Read the model definition and answer for the solid it produces. Units are mm, in the model's axes. A direction names the side the tool comes from. Round coordinates to 2 decimals unless told otherwise and drop trailing zeros. Loops run counter-clockwise (first coordinate to the right, second up) from the corner with the lowest first, then second, coordinate; pieces in that order, holes last. Notation, with made-up numbers: M -0.5,29 L 22.5,29 A26 cw 22.5,62 Z; hole C 23,1 d5. An arc over 180 degrees is marked long. Write each question's results on one line, items separated by ' | '.
Autodesk Inventor part; units mm, degrees
ref_plane "YZ Plane" through (0, 0, 0) normal (1, 0, 0) x (0, 1, 0)
ref_plane "XZ Plane" through (0, 0, 0) normal (0, 1, 0) x (-1, 0, 0)
ref_plane "XY Plane" through (0, 0, 0) normal (0, 0, 1) x (1, 0, 0)
sketch "Sketch1" plane through (0, 0, 0) normal (0, 0, 1) x (1, 0, 0)
  circle A0 centre (0, 0) radius 14
  circle A1 centre (0, 0) radius 20
  circle A2 centre (0, 0) radius 26
  circle A3 centre (0, 0) radius 31
  circle A4 centre (0, 0) radius 49
  circle A5 centre (0, 38.5) radius 7
  circle A6 centre (0, 38.5) radius 4
  dimension "d0" = 28
  dimension "d1" = 40
  dimension "d2" = 52
  dimension "d3" = 62
  dimension "d4" = 98
  dimension "d5" = 14
  dimension "d6" = 8
  dimension "d7" = 38.5
extrude "Extrusion1" add sketch "Sketch1" along normal blind 27.25 contours A0 | A1 | A2 | A3 | A4 | A5 | A6
extrude "Extrusion2" cut sketch "Sketch1" along normal through all contours A0
extrude "Extrusion3" cut sketch "Sketch1" along normal blind 7.25 contours A4 | A5 | A6
extrude "Extrusion4" cut sketch "Sketch1" along normal through all contours A6
extrude "Extrusion5" cut sketch "Sketch1" against normal blind 8 from surface at 27.25 contours A5
pattern_circular "Circular Pattern1" count 6 over 360 about axis through (0, 0, -10) along (0, 0, 1) of "Extrusion5", "Extrusion4"
extrude "Extrusion6" cut sketch "Sketch1" along normal blind 10 contours A0 | A1 | A2
extrude "Extrusion7" cut sketch "Sketch1" along normal blind 10 from surface at 10 contours A1
properties part number "B2"
Item 1: Straight lines are drawn through the part: line 1 (Y direction, x = 0, z = 23); line 2 (Y direction, x = 0, z = 13.5); line 3 (Y direction, x = -27.5, z = 21.25). For each, find the intervals that lie inside material, in ascending order.
Outcome:
line 1: y = -49 to -45.5, -31.5 to -14, 14 to 31.5, 45.5 to 49 | line 2: y = -49 to -42.5, -34.5 to -20, 20 to 34.5, 42.5 to 49 | line 3: y = -40.56 to -23.11, -15.39 to 15.39, 23.11 to 40.56
Item 2: The mould has two halves that part along Y. Classify faces 4 (the face through (-32, -15, 19.25)), 5 (the face through (26.34, -41.32, 17.11)), 6 (the face through (3, 35, 19.25)), 7 (the face through (10.2, -10.2, 27.25)): pulls with the +Y half, pulls with the -Y half, needs draft (parallel to the pull), parting line crosses it, or undercut.
Outcome:
face 4: undercut | face 5: parting line crosses it | face 6: undercut | face 7: needs draft
Item 3: The part is cut by section C-C (x = -9.5). Determine the outline of the cut face in (y, z), plus the area to 3 significant figures.
Outcome:
outline: M -48.07,7.25 L -29.51,7.25 L -29.51,0 L -24.2,0 L -24.2,10 L -17.6,10 L -17.6,20 L -10.28,20 L -10.28,27.25 L -48.07,27.25 Z; M 10.28,20 L 17.6,20 L 17.6,10 L 24.2,10 L 24.2,0 L 29.51,0 L 29.51,7.25 L 48.07,7.25 L 48.07,27.25 L 10.28,27.25 Z | area: 1,370 mm2
Item 4: Flat-ended cylindrical pins translate along their axes: pin 1 (6.5 mm diameter, centred on x = 33.34, y = 19.25, fed in from -Z); pin 2 (10 mm diameter, centred on x = 28, z = 4, fed in from -Y); pin 3 (9 mm diameter, centred on x = 33.34, y = -19.25, fed in from +Z); pin 4 (9 mm diameter, centred on x = -33.34, y = -19.25, fed in from -Z). Find the tip coordinate at first contact, or state that the pin passes through.
Outcome:
pin 1: passes through | pin 2: stops at y = -42.61 | pin 3: stops at z = 19.25 | pin 4: stops at z = 7.25
Item 5: For faces 1 (the face through (13.4, -15.3, 10)), 2 (the face through (-0.521, 34.534, 13.166)), 3 (the face through (-3, -35, 19.25)), determine the directions among +Z, -Z, +X, -X, +Y, -Y from which every point of the face is accessible in a straight line to the end or side of a thin tool.
Outcome:
face 1: -Z | face 2: +Z, -Z | face 3: +Z
Item 6: The part is cut by section A-A (y = 0). Determine the outline of the cut face in (x, z), plus the area to 3 significant figures.
Outcome:
outline: M -49,7.25 L -31,7.25 L -31,0 L -26,0 L -26,10 L -20,10 L -20,20 L -14,20 L -14,27.25 L -49,27.25 Z; M 14,20 L 20,20 L 20,10 L 26,10 L 26,0 L 31,0 L 31,7.25 L 49,7.25 L 49,27.25 L 14,27.25 Z | area: 1,290 mm2
Item 7: The part is cut by section D-D (z = 24.5). Determine the outline of the cut face in (x, y).
Outcome:
outline: C 0,0 d98; hole C -33.34,-19.25 d14; hole C -33.34,19.25 d14; hole C 0,0 d28; hole C 0,-38.5 d14; hole C 0,38.5 d14; hole C 33.34,-19.25 d14; hole C 33.34,19.25 d14
Item 8: The part is cut by section B-B (z = 3.25). Determine the outline of the cut face in (x, y), plus the area to 3 significant figures.
Outcome:
outline: C 0,0 d62; hole C 0,0 d52 | area: 895 mm2
